CAD build for the part. Positions are in the model's coordinates, mm. A direction names the side the tool comes from. Round coordinates to 2 decimals unless told otherwise and drop trailing zeros. Loops run counter-clockwise (first coordinate to the right, second up) from the corner with the lowest first, then second, coordinate; pieces in that order, holes last. Notation, with made-up numbers: M 67,78 L 126,78 A5 ccw 126,87 Z; hole C -31,-13.5 d8. An arc over 180 degrees is marked long. Use a Markdown table: item, result. Add a question column.
(1) Flat gauge pins, fed straight in: P1, Ø1.5, axis at y = -41.5, z = 0.5, coming from the +X side; P2, Ø1.5, axis at x = 16.5, z = 1, coming from the +Y side. Where does each tip first touch, or does it go through?
(2) Band-saw the part on A-A, the plane y = 24.5. Write the cut outline in (x, z).
(3) Wall check: L1, parallel to Y at x = -1, z = 0.5; L2, parallel to X at y = 14, z = 0.25; L3, parallel to Y at x = 37.5, z = 2.45. Give the ranges that are in metal, low to high.
(4) Two-plate mould, pull along X, no slides. Class faces 1 (the face through (-40.52, -85.15, 1.52)), 2 (the face through (0, -86.3, 2)), 3 (the face through (40.65, -85.02, 1.52)), 4 (the face through (1, 1, 3)): released by +X, released by -X, zero draft, split by the parting line, or undercut.
(5) Which spindle directions (+Z, -Z, +X, -X, +Y, -Y) get a long thin tool onto all of the face, cutting with end or side? Do faces 5 (the face through (-41.8, -1, 2)), 6 (the face through (41.8, 1, 2)), 7 (the face through (29, -87.4, 2)), 8 (the face through (0, 86.3, 2)). Say none if no direction does.
from build123d import *

# Parameters (mm, degrees)
BOSS_EXTRUDE1_DEPTH = 3


with BuildPart() as part:
    # Sketch1 → Boss-Extrude1 (new body)
    with BuildSketch(Plane.XY.offset(3)):
        with BuildLine():
            Line((42.4, 57.4), (42.3, 57.4))
            ThreePointArc((42.3, 57.4), (41.946446609, 57.253553391), (41.8, 56.9))
            Line((41.8, 56.9), (41.8, -56.9))
            ThreePointArc((41.8, -56.9), (41.946446609, -57.253553391), (42.3, -57.4))
            Line((42.3, -57.4), (42.4, -57.4))
            ThreePointArc((42.4, -57.4), (42.753553391, -57.546446609), (42.9, -57.9))
            Line((42.9, -57.9), (42.9, -79.5))
            ThreePointArc((42.9, -79.5), (40.586143571, -85.086143571), (35, -87.4))
            Line((35, -87.4), (23.4, -87.4))
            ThreePointArc((23.4, -87.4), (23.046446609, -87.253553391), (22.9, -86.9))
            Line((22.9, -86.9), (22.9, -86.8))
            ThreePointArc((22.9, -86.8), (22.753553391, -86.446446609), (22.4, -86.3))
            Line((22.4, -86.3), (-22.4, -86.3))
            ThreePointArc((-22.4, -86.3), (-22.753553391, -86.446446609), (-22.9, -86.8))
            Line((-22.9, -86.8), (-22.9, -86.9))
            ThreePointArc((-22.9, -86.9), (-23.046446609, -87.253553391), (-23.4, -87.4))
            Line((-23.4, -87.4), (-35, -87.4))
            ThreePointArc((-35, -87.4), (-40.586143571, -85.086143571), (-42.9, -79.5))
            Line((-42.9, -79.5), (-42.9, -57.9))
            ThreePointArc((-42.9, -57.9), (-42.753553391, -57.546446609), (-42.4, -57.4))
            Line((-42.4, -57.4), (-42.3, -57.4))
            ThreePointArc((-42.3, -57.4), (-41.946446609, -57.253553391), (-41.8, -56.9))
            Line((-41.8, -56.9), (-41.8, 56.9))
            ThreePointArc((-41.8, 56.9), (-41.946446609, 57.253553391), (-42.3, 57.4))
            Line((-42.3, 57.4), (-42.4, 57.4))
            ThreePointArc((-42.4, 57.4), (-42.753553391, 57.546446609), (-42.9, 57.9))
            Line((-42.9, 57.9), (-42.9, 79.5))
            ThreePointArc((-42.9, 79.5), (-40.586143571, 85.086143571), (-35, 87.4))
            Line((-35, 87.4), (-23.4, 87.4))
            ThreePointArc((-23.4, 87.4), (-23.046446609, 87.253553391), (-22.9, 86.9))
            Line((-22.9, 86.9), (-22.9, 86.8))
            ThreePointArc((-22.9, 86.8), (-22.753553391, 86.446446609), (-22.4, 86.3))
            Line((-22.4, 86.3), (22.4, 86.3))
            ThreePointArc((22.4, 86.3), (22.753553391, 86.446446609), (22.9, 86.8))
            Line((22.9, 86.8), (22.9, 86.9))
            ThreePointArc((22.9, 86.9), (23.046446609, 87.253553391), (23.4, 87.4))
            Line((23.4, 87.4), (35, 87.4))
            ThreePointArc((35, 87.4), (40.586143571, 85.086143571), (42.9, 79.5))
            Line((42.9, 79.5), (42.9, 57.9))
            ThreePointArc((42.9, 57.9), (42.753553391, 57.546446609), (42.4, 57.4))
        make_face()
    extrude(amount=-BOSS_EXTRUDE1_DEPTH)


solid = part.part
Return value:
| question | item | result |
|---|---|---|
| 1 | P1 | x = 41.8 |
| 1 | P2 | y = 86.3 |
| 2 | outline | M -41.8,0 L 41.8,0 L 41.8,3 L -41.8,3 Z |
| 3 | L1 | -86.3 to 86.3 |
| 3 | L2 | -41.8 to 41.8 |
| 3 | L3 | -86.99 to 86.99 |
| 4 | face 1 | released by -X |
| 4 | face 2 | undercut |
| 4 | face 3 | released by +X |
| 4 | face 4 | zero draft |
| 5 | face 5 | +Z, -Z, -X |
| 5 | face 6 | +Z, -Z, +X |
| 5 | face 7 | +Z, -Z, +X, -X, -Y |
| 5 | face 8 | +Z, -Z, +Y |
